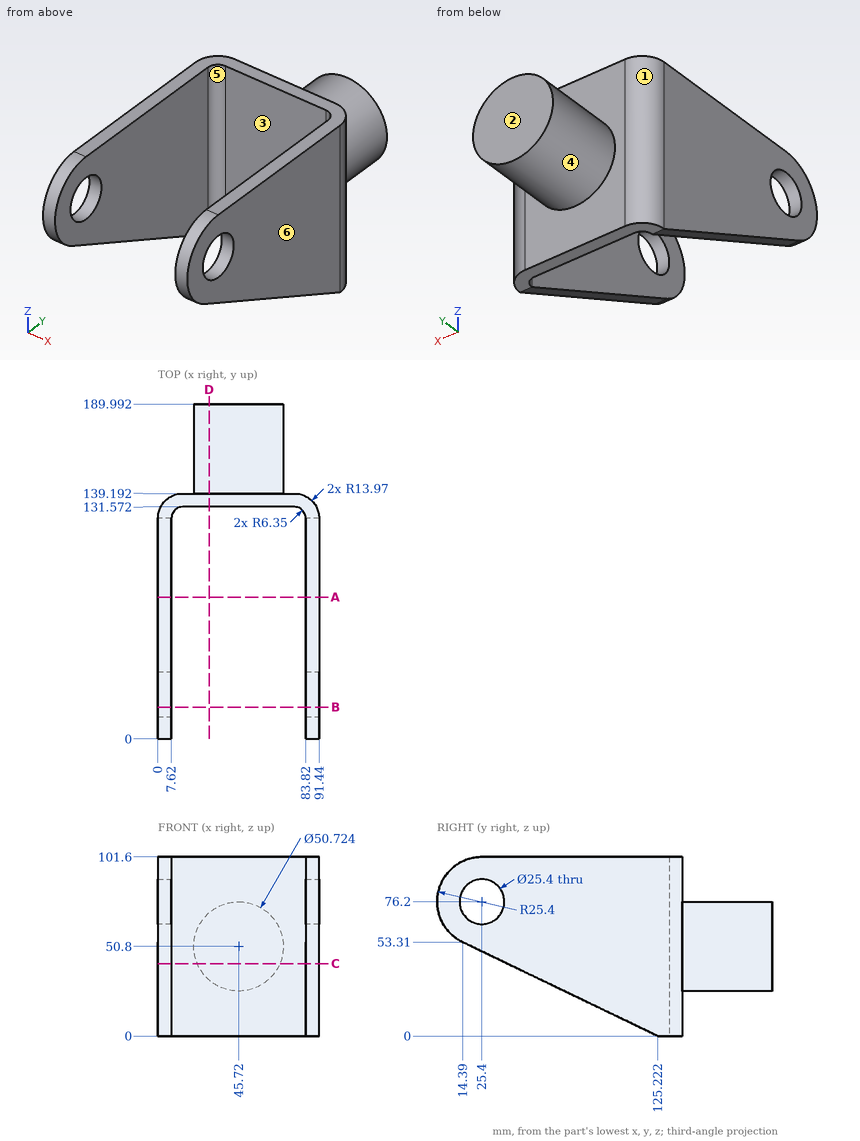
Input: dimensioned drawing with shaded views. Units: mm. Origin: part minimum x, y, z. A direction names the side the tool comes from. Round coordinates to 2 decimals unless told otherwise and drop trailing zeros. Order: outer loops, then holes, each group sorted by start corner. A loop starts at its lowest first (then second) coordinate and runs counter-clockwise, first axis right, second up. Notation, with made-up numbers: (3.25, -2) - (41.25, -2) arc R33 cw to (41.25, 31) - close; hole circle Ø9 at (70.25, 4). An arc over 180 degrees is marked (long way). Write item = value, one per line. Start each with the question number.
Q1. Pin query (flat end, axial travel): pin 1 (5 mm diameter, centred on x = 45, z = 23.5, fed in from -Y); pin 2 (15 mm diameter, centred on y = 25.4, z = 76.2, fed in from -X); pin 3 (5 mm diameter, centred on x = 20, z = 37, fed in from +Y). Return the tip coordinate at first contact, or that it passes through.
Q2. Pull-direction query (X, two-part tool) for the marked faces 1, 2 and 3; classes: +X half, -X half, draft (parallel to the pull), parting line (faces both ways), or undercut.
Q3. Cut plane A-A on y = 80.5. Return the cut outline in (x, z), and give its area (3 significant figures).
Q4. Cut plane B-B on y = 18. Return the cut outline in (x, z).
Q5. Cut plane C-C on z = 41. Return the cut outline in (x, y).
Q6. Cut plane D-D on x = 29. Return the cut outline in (y, z).
Q7. Ray query, line 1 (X direction, y = 91, z = 29.5); line 2 (Y direction, x = 46, z = 34); line 3 (Y direction, x = 40, z = 6.5). Return the intervals inside material, ascending. Write a range as from..to.
Q8. Access query for the marked faces 4, 5 and 6. Directions: +Z, -Z, +X, -X, +Y, -Y. A direction counts if a zero-diameter tool reaches every point of the face in a straight line with its end or side. Return the directions, or none.
Outcome:
q1.pin_1 = 131.57
q1.pin_2 = through
q1.pin_3 = 139.19
q2.face_1 = -X half
q2.face_2 = draft
q2.face_3 = undercut
q3.outline = (0, 21.51) - (7.62, 21.51) - (7.62, 101.6) - (0, 101.6) - close; (83.82, 21.51) - (91.44, 21.51) - (91.44, 101.6) - (83.82, 101.6) - close
q3.area = 1,220 mm^2
q4.outline = (0, 51.57) - (7.62, 51.57) - (7.62, 65.88) - (0, 65.88) - close; (0, 86.52) - (7.62, 86.52) - (7.62, 100.5) - (0, 100.5) - close; (83.82, 51.57) - (91.44, 51.57) - (91.44, 65.88) - (83.82, 65.88) - close; (83.82, 86.52) - (91.44, 86.52) - (91.44, 100.5) - (83.82, 100.5) - close
q5.outline = (0, 39.98) - (7.62, 39.98) - (7.62, 125.22) arc R6.35 cw to (13.97, 131.57) - (77.47, 131.57) arc R6.35 cw to (83.82, 125.22) - (83.82, 39.98) - (91.44, 39.98) - (91.44, 125.22) arc R13.97 ccw to (77.47, 139.19) - (69.11, 139.19) - (69.11, 189.99) - (22.33, 189.99) - (22.33, 139.19) - (13.97, 139.19) arc R13.97 ccw to (0, 125.22) - close
q6.outline = (131.57, 0) - (139.19, 0) - (139.19, 31.73) - (189.99, 31.73) - (189.99, 69.87) - (139.19, 69.87) - (139.19, 101.6) - (131.57, 101.6) - close
q7.line_1 = 0..7.62, 83.82..91.44
q7.line_2 = 131.57..189.99
q7.line_3 = 131.57..139.19
q8.face_4 = +Y
q8.face_5 = +Z, -Z, -Y
q8.face_6 = +Z, -Z, +X, +Y, -Y
